Input: part model. Units: mm. Frame: model coordinates. A direction names the side the tool comes from. Coordinates: 2 decimals unless noted, no trailing zeros. Order: outer loops, then holes, each group sorted by start corner. A loop starts at its lowest first (then second) coordinate and runs counter-clockwise, first axis right, second up. Notation, with made-up numbers: (80, -25) -> (107, -25) arc R35 cw to (107, 11) -> close; hole circle Ø9 at (0.25, 71.5). An arc over 180 degrees is marked (long way). Answer as CSV lines item,"result".
from build123d import *

# Parameters (mm, degrees)
SKETCH1_W                 = 50
SKETCH1_H                 = 8
BOSS_EXTRUDE1_DEPTH       = 3
F_8_CLEARANCE_HOLE1_D     = 4.4958
F_8_CLEARANCE_HOLE1_DEPTH = 17
F_8_CLEARANCE_HOLE1_TIP   = 1.350674586
SKETCH3_W                 = 50
SKETCH3_H                 = 3
BOSS_EXTRUDE2_DEPTH       = 10
SKETCH5_W                 = 46
SKETCH5_H                 = 8
BOSS_EXTRUDE3_DEPTH       = 150
SKETCH6_R                 = 0.5207
CUT_EXTRUDE1_DEPTH        = 30


with BuildPart() as part:
    # Sketch1 → Boss-Extrude1 (new body)
    with BuildSketch(Plane(origin=(0, 0, 0), x_dir=(1, 0, 0), z_dir=(0, 1, 0))):
        with Locations((17.773632998, 0.313559322)):
            Rectangle(SKETCH1_W, SKETCH1_H)
    extrude(amount=BOSS_EXTRUDE1_DEPTH)

    # #8 Clearance Hole1
    with Locations(Plane(origin=(0.523632998, 3, -0.313559322), x_dir=(0, 0, 1), z_dir=(0, 1, 0))):
        with Locations((0, 0), (0, 34.5)):
            Hole(F_8_CLEARANCE_HOLE1_D / 2, depth=F_8_CLEARANCE_HOLE1_DEPTH)
            with Locations((0, 0, -(F_8_CLEARANCE_HOLE1_DEPTH + F_8_CLEARANCE_HOLE1_TIP / 2))):  # 118° drill point
                Cone(0, F_8_CLEARANCE_HOLE1_D / 2, F_8_CLEARANCE_HOLE1_TIP, mode=Mode.SUBTRACT)

    # Sketch3 → Boss-Extrude2 (add)
    with BuildSketch(Plane(origin=(0, 0, -4.313559322), x_dir=(-1, 0, 0), z_dir=(0, 0, -1))):
        with Locations((-17.773632998, 1.5)):
            Rectangle(SKETCH3_W, SKETCH3_H)
    extrude(amount=BOSS_EXTRUDE2_DEPTH)

    # Sketch5 → Boss-Extrude3 (add)
    with BuildSketch(Plane(origin=(0, 3, 0), x_dir=(1, 0, 0), z_dir=(0, 1, 0))):
        with Locations((17.773632998, 10.313559322)):
            Rectangle(SKETCH5_W, SKETCH5_H)
    extrude(amount=BOSS_EXTRUDE3_DEPTH)

    # Sketch6 → Cut-Extrude1 (cut)
    with BuildSketch(Plane(origin=(0, 153, 0), x_dir=(1, 0, 0), z_dir=(0, 1, 0))):
        with Locations((17.773632998, 13.063559322)):
            Circle(SKETCH6_R)
    extrude(amount=-CUT_EXTRUDE1_DEPTH, mode=Mode.SUBTRACT)


solid = part.part
1. Mould query, pull axis Z, two halves, no side actions, for faces 4 (the face through (36.92, 1.48, -1.52)), 5 (the face through (-0.844, 1.479, 1.47)), 6 (the face through (42.774, 1, -5)), 7 (the face through (17, 77, -6.314)). Classes: released by +Z, released by -Z, zero draft, split by the parting line, or undercut.
Findings:
face 4,"undercut"
face 5,"undercut"
face 6,"zero draft"
face 7,"released by +Z"
2. Cut plane A-A (z = -1.25). Return the cut outline in (x, y).
Findings:
outline,"(-7.23, 0) -> (-1.52, 0) -> (-1.52, 3) -> (-7.23, 3) -> close; (2.57, 0) -> (32.98, 0) -> (32.98, 3) -> (2.57, 3) -> close; (37.07, 0) -> (42.77, 0) -> (42.77, 3) -> (37.07, 3) -> close"
3. Ray query, line 1 along Y through (x, z) = (11.5, 3); line 2 along X through (y, z) = (59.5, -12.25); line 3 along Z through (x, y) = (25, 37.5). Return the intervals inside material, ascending.
Findings:
line 1,"y = 0 to 3"
line 2,"x = -5.23 to 40.77"
line 3,"z = -14.31 to -6.31"
4. Reachability of faces 1 (the face through (40.774, 77, -10)), 2 (the face through (-7.226, 1, -5)), 3 (the face through (-5.226, 77, -10)) from +Z, -Z, +X, -X, +Y, -Y: full face, straight path, thin tool, end or side. Return the list, or none.
Findings:
face 1,"+Z, -Z, +X, +Y"
face 2,"+Z, -Z, -X, +Y, -Y"
face 3,"+Z, -Z, -X, +Y"
5. Cut plane D-D (z = -9.25). Return the cut outline in (x, y), plus the area to 3 significant figures.
Findings:
outline,"(-7.23, 0) -> (42.77, 0) -> (42.77, 3) -> (40.77, 3) -> (40.77, 153) -> (-5.23, 153) -> (-5.23, 3) -> (-7.23, 3) -> close"
area,"7,050 mm2"
6. Contact query for flat-ended pins moving along their axis: pin 1 (6.5 mm diameter, centred on y = 67, z = -9.5, fed in from -X); pin 2 (0.8 mm diameter, centred on x = 17.77, z = -13.06, fed in from +Y); pin 3 (4 mm diameter, centred on x = 20.5, z = -4, fed in from +Y); pin 4 (3.5 mm diameter, centred on x = 35.02, z = -0.31, fed in from -Y). Output: stop coordinate, or through.
Findings:
pin 1,"stops at x = -5.23"
pin 2,"stops at y = 123"
pin 3,"stops at y = 3"
pin 4,"passes through"
7. Cut plane B-B (x = 10.5). Return the cut outline in (y, z), plus the area to 3 significant figures.
Findings:
outline,"(0, -14.31) -> (153, -14.31) -> (153, -6.31) -> (3, -6.31) -> (3, 3.69) -> (0, 3.69) -> close"
area,"1,250 mm2"
8. Cut plane C-C (y = 133). Return the cut outline in (x, z).
Findings:
outline,"(-5.23, -14.31) -> (40.77, -14.31) -> (40.77, -6.31) -> (-5.23, -6.31) -> close; hole circle Ø1.04 at (17.77, -13.06)"
